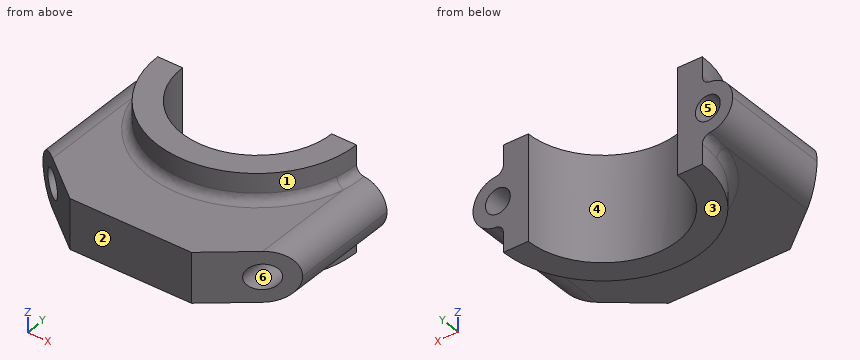
```python
from build123d import *

# Parameters (mm, degrees)
BOSS_EXTRUDE1_DEPTH    = 19
BOSS_EXTRUDE2_DEPTH    = 9
FILLET1_START          = -60
FILLET1_DEPTH          = 60
FILLET2_START          = -60
FILLET2_DEPTH          = 60
M10X1_5_TAPPED_HOLE1_D = 9
FILLET3_R              = 3


with BuildPart() as part:
    # Sketch1 → Boss-Extrude1 (new, symmetric)
    with BuildSketch(Plane.XY):
        with BuildLine():
            Line((-27, 0), (-36, 0))
            ThreePointArc((-36, 0), (0, -36), (36, 0))
            Line((36, 0), (27, 0))
            ThreePointArc((27, 0), (0, -27), (-27, 0))
        make_face()
    extrude(amount=BOSS_EXTRUDE1_DEPTH, both=True)

    # Sketch1<3> → Boss-Extrude2 (add, symmetric)
    with BuildSketch(Plane.XY):
        with BuildLine():
            Line((-36, 0), (-47, 0))
            Line((-47, 0), (-47, -40))
            Line((-47, -40), (-22, -60))
            Line((-22, -60), (22, -60))
            Line((22, -60), (47, -40))
            Line((47, -40), (47, 0))
            Line((47, 0), (36, 0))
            ThreePointArc((36, 0), (0, -36), (-36, 0))
        make_face()
    extrude(amount=BOSS_EXTRUDE2_DEPTH, both=True)

    # Fillet1: read off the stored shape, not the designer's step
    # Fillet1 outline → Fillet1 (cut)
    with BuildSketch(Plane(origin=(0, 0, 0), x_dir=(1, 0, 0), z_dir=(0, 1, 0)).offset(FILLET1_START)):
        with BuildLine():
            Line((47, 9), (38, 9))
            ThreePointArc((38, 9), (44.363961031, 6.363961031), (47, 0))
            Line((47, 0), (47, 9))
        make_face()
        with BuildLine():
            Line((47, -9), (47, 0))
            ThreePointArc((47, 0), (44.363961031, -6.363961031), (38, -9))
            Line((38, -9), (47, -9))
        make_face()
    extrude(amount=FILLET1_DEPTH, mode=Mode.SUBTRACT)

    # Fillet2: read off the stored shape, not the designer's step
    # Fillet2 outline → Fillet2 (cut)
    with BuildSketch(Plane(origin=(0, 0, 0), x_dir=(1, 0, 0), z_dir=(0, 1, 0)).offset(FILLET2_START)):
        with BuildLine():
            Line((-47, -9), (-38, -9))
            ThreePointArc((-38, -9), (-44.363961031, -6.363961031), (-47, 0))
            Line((-47, 0), (-47, -9))
        make_face()
        with BuildLine():
            Line((-47, 9), (-47, 0))
            ThreePointArc((-47, 0), (-44.363961031, 6.363961031), (-38, 9))
            Line((-38, 9), (-47, 9))
        make_face()
    extrude(amount=FILLET2_DEPTH, mode=Mode.SUBTRACT)

    # M10x1.5 Tapped Hole1 (through all)
    with Locations(Plane(origin=(-38, 0, 0), x_dir=(0, 0, 1), z_dir=(0, 1, 0))):
        with Locations((0, 0), (0, 76)):
            Hole(M10X1_5_TAPPED_HOLE1_D / 2)

    # Fillet3
    fillet3_edges = [part.edges().sort_by_distance(p)[0] for p in [
        (0, -36, -9),
        (0, -36, 9),
    ]]
    fillet(fillet3_edges, radius=FILLET3_R)


solid = part.part
```
Check sheet for the modelled part. Datum: model origin and axes. Units: mm. Face numbers are marked on the shaded views. A direction names the side the tool comes from. Round coordinates to 2 decimals unless told otherwise and drop trailing zeros. Order: outer loops, then holes, each group sorted by start corner. A loop starts at its lowest first (then second) coordinate and runs counter-clockwise, first axis right, second up. Notation, with made-up numbers: (70, 43) - (86, 43) arc R13 cw to (86, 64) - close; hole circle Ø2 at (32, 15). An arc over 180 degrees is marked (long way). Answer as CSV lines item,"result". Start each with the question number.
1) Depth check by flat-ended pin: pin 1 (1.5 mm diameter, centred on y = -42.5, z = 1.5, fed in from +X); pin 2 (8 mm diameter, centred on y = -47, z = 5, fed in from +X); pin 3 (2 mm diameter, centred on x = -11, y = -49.5, fed in from -Z). Enter the tip coordinate at first touch or a pass-through.
2) Draft check along Z on the marked faces 3, 4, 5 and 6. Enter one of: +Z half, -Z half, draft (parallel to the pull), parting line (faces both ways), or undercut.
3) Tool access check on the marked faces 1 and 2. Record the directions out of +Z, -Z, +X, -X, +Y, -Y that give a thin tool (end or side, any length) a straight path to the whole face; none if there is none.
4) Section check B-B (y = -19). Give the number of separate pieces and of enclosed holes in the cut face, then the cut area to 3 significant figures.
5) Section check C-C (z = -7). Record the cut outline in (x, y).
6) Section check A-A (z = 1). Record the cut outline in (x, y).
7) Scan lines: probe 1 along Z at (x, y) = (38, -38); probe 2 along X at (y, z) = (-3, -3); probe 3 along X at (y, z) = (-5, -10). Record each from-to range of solid material in increasing order.
Determined:
1,pin 1,"x = 44.81"
1,pin 2,"x = 43.25"
1,pin 3,"z = -9"
2,face 3,"-Z half"
2,face 4,"draft"
2,face 5,"undercut"
2,face 6,"undercut"
3,face 1,"+Z, -Y"
3,face 2,"+Z, -Z, +X, -X, -Y"
4,separate pieces,"2"
4,enclosed holes,"2"
4,area,"1,270 mm^2"
5,outline,"(-43.66, -42.67) - (-22, -60) - (22, -60) - (43.66, -42.67) - (43.66, 0) - (27, 0) arc R27 cw to (-27, 0) - (-43.66, 0) - close"
6,outline,"(-46.94, -40.04) - (-42.39, -43.69) - (-42.39, 0) - (-46.94, 0) - close; (-33.61, -50.71) - (-22, -60) - (22, -60) - (33.61, -50.71) - (33.61, 0) - (27, 0) arc R27 cw to (-27, 0) - (-33.61, 0) - close; (42.39, -43.69) - (46.94, -40.04) - (46.94, 0) - (42.39, 0) - close"
7,probe 1,"-9 to -4.5, 4.5 to 9"
7,probe 2,"-46.49 to -41.35, -34.65 to -26.83, 26.83 to 34.65, 41.35 to 46.49"
7,probe 3,"-36.41 to -26.53, 26.53 to 36.41"
